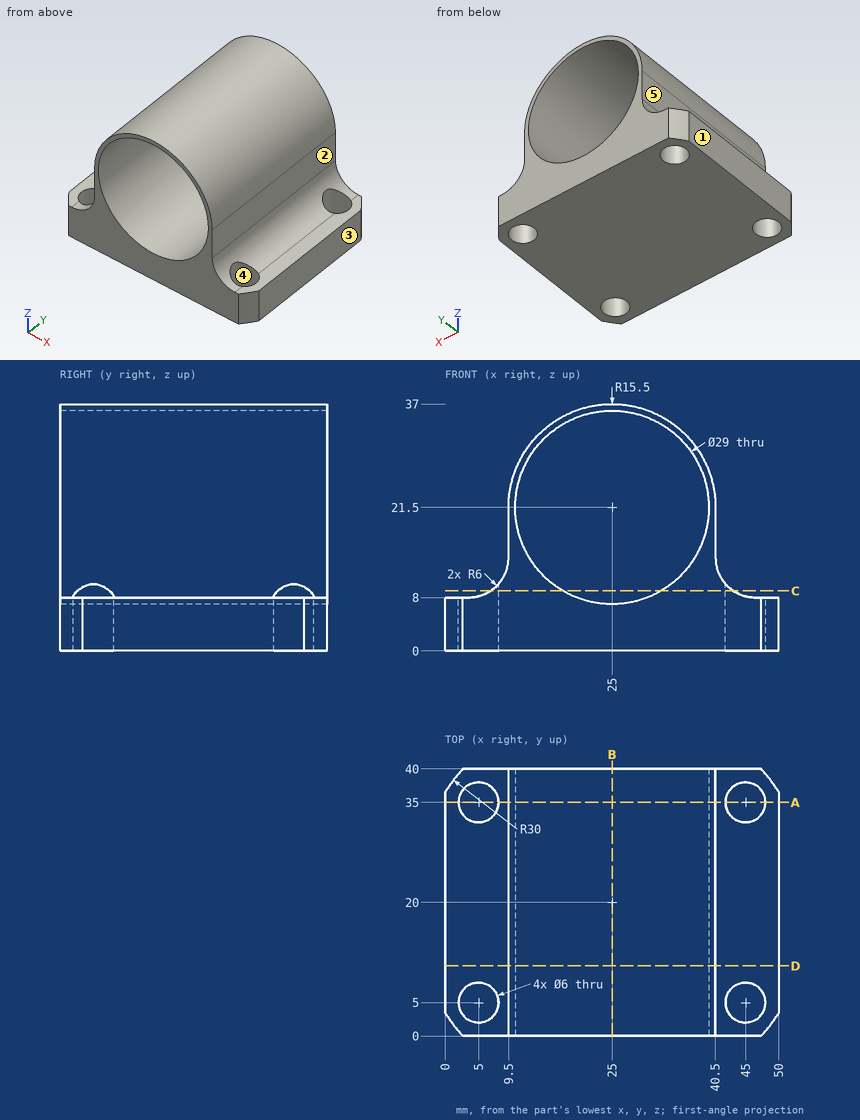
For this review, use the dimensioned drawing (mm, ordinates from the lowest corner) and the shaded views. A direction names the side the tool comes from. Round coordinates to 2 decimals unless told otherwise and drop trailing zeros. Write each loop counter-clockwise with the first axis right and the second up, starting at its lowest first coordinate (ties: lowest second). Pieces come first, ordered by that corner, then holes. Notation, with made-up numbers: (20.5, -1.5) -> (47.5, -1.5) arc R9 cw to (47.5, 14.5) -> close; hole circle Ø6 at (50.25, 11.5). An arc over 180 degrees is marked (long way). One line per item, written item: value. Start each with the question number.
Q1. To check wall thickness, follow probe 1 along Y at (x, z) = (5, 7); probe 2 along X at (y, z) = (3.5, 33); probe 3 along X at (y, z) = (36.5, 16). State the ranges of each line that lie inside material, in increasing order.
Q2. Tool access review of the marked faces 1 and 2: name each direction out of +Z, -Z, +X, -X, +Y, -Y from which nothing blocks a thin tool from reaching the whole face with its end or side.
Q3. Add section D-D (y = 10.5). Give the boundary of the cut face in (x, z), then the cut area to 3 significant figures.
Q4. Add section B-B (x = 25). Give the boundary of the cut face in (y, z), then the cut area to 3 significant figures.
Q5. Add section C-C (z = 9). Give the boundary of the cut face in (x, y), then the cut area to 3 significant figures.
Q6. The part is to be moulded in two halves that separate along X. For the marked faces 3, 4 and 5, say which applies: pulls with the +X half, pulls with the -X half, needs draft (parallel to the pull), parting line crosses it, or undercut.
Q7. Insertion check: P1, Ø6, axis at x = 33, y = 25, coming from the +Z side; P2, Ø4, axis at y = 12.5, z = 18.5, coming from the -X side; P3, Ø4, axis at x = 25.5, y = 5.5, coming from the +Z side; P4, Ø4, axis at x = 49, y = 29, coming from the +Z side. Each pin has a flat end and moves straight along its axis. Give the tip position at first contact, or say it passes through.
Q8. Add section A-A (y = 35). Give the boundary of the cut face in (x, z).
Response:
1. probe 1: y = 0 to 2, 8 to 32, 38 to 40
1. probe 2: x = 14.61 to 16.17, 33.83 to 35.39
1. probe 3: x = 9.5 to 11.58, 38.42 to 40.5
2. face 1: +Z, -Z, -X, +Y, -Y
2. face 2: +Z, +X, +Y, -Y
3. outline: (0, 0) -> (50, 0) -> (50, 8) -> (46.5, 8) arc R6 cw to (40.5, 14) -> (40.5, 21.5) arc R15.5 ccw to (9.5, 21.5) -> (9.5, 14) arc R6 cw to (3.5, 8) -> (0, 8) -> close; hole circle Ø29 at (25, 21.5)
3. area: 551 mm^2
4. outline: (0, 0) -> (40, 0) -> (40, 7) -> (0, 7) -> close; (0, 36) -> (40, 36) -> (40, 37) -> (0, 37) -> close
4. area: 320 mm^2
5. outline: (6.82, 0) -> (17.65, 0) -> (17.65, 40) -> (6.82, 40) -> (6.82, 37.39) arc R3 cw to (6.82, 32.61) -> (6.82, 7.39) arc R3 cw to (6.82, 2.61) -> close; (32.35, 0) -> (43.18, 0) -> (43.18, 2.61) arc R3 cw to (43.18, 7.39) -> (43.18, 32.61) arc R3 cw to (43.18, 37.39) -> (43.18, 40) -> (32.35, 40) -> close
5. area: 851 mm^2
6. face 3: pulls with the +X half
6. face 4: undercut
6. face 5: pulls with the -X half
7. P1: stops at z = 36.17
7. P2: stops at x = 9.5
7. P3: stops at z = 37
7. P4: stops at z = 8
8. outline: (0, 0) -> (2, 0) -> (2, 8) -> (0, 8) -> close; (8, 0) -> (42, 0) -> (42, 10.03) arc R6 cw to (40.5, 14) -> (40.5, 21.5) arc R15.5 ccw to (9.5, 21.5) -> (9.5, 14) arc R6 cw to (8, 10.03) -> close; (48, 0) -> (50, 0) -> (50, 8) -> (48, 8) -> close; hole circle Ø29 at (25, 21.5)
